```python
from build123d import *

# Parameters (mm, degrees)
F0_R      = 37.5
F1_DEPTH  = 69.5
F2_R      = 30
F3_DEPTH  = 31
F4_R      = 29.5
F5_DEPTH  = 99.5
F7_DEPTH  = 75
F10_R     = 7
F11_DEPTH = 67.001


with BuildPart() as f1:
    # F0 (on Front) → F1 (new body, symmetric)
    with BuildSketch(Plane.XZ):
        Circle(F0_R)
    extrude(amount=F1_DEPTH, both=True)

    # F2 (on face) → F3 (join)
    with BuildSketch(Plane.XZ.offset(69.5)):
        Circle(F2_R)
    extrude(amount=F3_DEPTH)

    # F4 (on face) → F5 (join)
    with BuildSketch(Plane.XZ.offset(100.5)):
        Circle(F4_R)
    extrude(amount=F5_DEPTH)

    # F6 (on face) → F7 (cut)
    with BuildSketch(Plane.XZ.offset(200)):
        with BuildLine():
            Line((19.653244007, -22), (-19.653244007, -22))
            ThreePointArc((-19.653244007, -22), (0, -29.5), (19.653244007, -22))
        make_face()
    extrude(amount=-F7_DEPTH, mode=Mode.SUBTRACT)

    # F10 (on plane+point) → F11 (cut, through all)
    with BuildSketch(Plane.XY.offset(29.5)):
        with Locations((0, -170)):
            Circle(F10_R)
    extrude(amount=-F11_DEPTH, mode=Mode.SUBTRACT)

    # F12: F1 across plane


with BuildPart() as f1_1:
    add(f1.part)
    add(f1.part.mirror(Plane.XZ))


solid = f1_1.part
```
Design review of the part built by this model. Coordinates are the model's own, in mm. A direction names the side the tool comes from. Round coordinates to 2 decimals unless told otherwise and drop trailing zeros. Write each loop counter-clockwise with the first axis right and the second up, starting at its lowest first coordinate (ties: lowest second). Pieces come first, ordered by that corner, then holes.
Item 1: The part is to be moulded in two halves that separate along Y. For faces 6 (the cylindrical face through (-1.517, -176.834, 4.112)), 7 (the cylindrical face through (-4.88, -0.97, 37.18)), 8 (the flat face through (0, 200, 4)), 9 (the cylindrical face through (-1.517, 176.834, 4.112)), say which applies: +Y half, -Y half, draft (parallel to the pull), parting line (faces both ways), or undercut.
Item 2: We need section C-C on y = -80.5. Write out the cut boundary in (x, z), and give its area (3 significant figures).
Item 3: We need section A-A on z = 0. Write out the cut boundary in (x, y), and give its area (3 significant figures).
Item 4: Clearance check with flat-ended pins moving along their axes: pin 1 Ø3.5 at (x, z) = (-7.5, -24.5) entering from -Y; pin 2 Ø12 at (x, y) = (-7, 145.5) entering from -Z; pin 3 Ø2 at (x, z) = (-3.5, -27) entering from +Y. State where each tip first meets the part, or that it passes through.
Item 5: We need section D-D on z = 16.5. Write out the cut boundary in (x, y), and give its area (3 significant figures).
Item 6: We need section B-B on y = 170. Write out the cut boundary in (x, z), and give its area (3 significant figures).
Item 7: For faces 1 (the flat face through (-17, 69.5, 25)), 2 (the flat face through (0, 125, -25)), 3 (the flat face through (0, -200, 4)), 4 (the cylindrical face through (-3.84, -149.55, 29.25)), 5 (the flat face through (5, -163, -22)), list the 3-axis set-ups (+Z, -Z, +X, -X, +Y, -Y) from which the entire face can be reached by the end or side of a thin tool; tool diameter is ignored.
Item 8: For probe 1 along Y at (x, z) = (0, 19); probe 2 along X at (y, z) = (-170, -1); probe 3 along X at (y, z) = (170, 9), list the stretches that pass through material, from the lowest coordinate up.
Returned:
1. face 6: undercut
1. face 7: draft
1. face 8: +Y half
1. face 9: undercut
2. outline: circle Ø60 at (0, 0)
2. area: 2,830 mm2
3. outline: (-37.5, -69.5) - (-30, -69.5) - (-30, -100.5) - (-29.5, -100.5) - (-29.5, -200) - (29.5, -200) - (29.5, -100.5) - (30, -100.5) - (30, -69.5) - (37.5, -69.5) - (37.5, 69.5) - (30, 69.5) - (30, 100.5) - (29.5, 100.5) - (29.5, 200) - (-29.5, 200) - (-29.5, 100.5) - (-30, 100.5) - (-30, 69.5) - (-37.5, 69.5) - close; hole circle Ø14 at (0, -170); hole circle Ø14 at (0, 170)
3. area: 25,600 mm2
4. pin 1: stops at y = -125
4. pin 2: stops at z = -22
4. pin 3: stops at y = 125
5. outline: (-33.67, -69.5) - (-25.05, -69.5) - (-25.05, -100.5) - (-24.45, -100.5) - (-24.45, -200) - (24.45, -200) - (24.45, -100.5) - (25.05, -100.5) - (25.05, -69.5) - (33.67, -69.5) - (33.67, 69.5) - (25.05, 69.5) - (25.05, 100.5) - (24.45, 100.5) - (24.45, 200) - (-24.45, 200) - (-24.45, 100.5) - (-25.05, 100.5) - (-25.05, 69.5) - (-33.67, 69.5) - close; hole circle Ø14 at (0, -170); hole circle Ø14 at (0, 170)
5. area: 21,900 mm2
6. outline: (-19.65, -22) - (-7, -22) - (-7, 28.66) arc R29.5 ccw to start; (7, -22) - (19.65, -22) arc R29.5 ccw to (7, 28.66) - close
6. area: 1,810 mm2
7. face 1: +Y
7. face 2: -Z, +X, -X, +Y
7. face 3: +Z, -Z, +X, -X, -Y
7. face 4: -Y
7. face 5: -Z, +X, -X, -Y
8. probe 1: y = -200 to -177, -163 to 163, 177 to 200
8. probe 2: x = -29.48 to -7, 7 to 29.48
8. probe 3: x = -28.09 to -7, 7 to 28.09
